```python
from build123d import *

# Parameters (mm, degrees)
F0_R     = 1
F0_R_2   = 0.5
F1_DEPTH = 4.2
F3_DEPTH = 3.2
F4_R     = 1.85
F4_R_2   = 1
F5_DEPTH = 2.2


with BuildPart() as f1:
    # F0 (on Top) → F1 (new body)
    with BuildSketch(Plane.XY):
        with BuildLine():
            Line((-1.99505, 12.940625), (-2.892823, 0.203906))
            ThreePointArc((-2.892823, 0.203906), (0, -2.9), (2.892823, 0.203906))
            Line((2.892823, 0.203906), (1.99505, 12.940625))
            ThreePointArc((1.99505, 12.940625), (0, 14.8), (-1.99505, 12.940625))
        make_face()
        Circle(F0_R, mode=Mode.SUBTRACT)
        with Locations((0, 4.8)):
            Circle(F0_R_2, mode=Mode.SUBTRACT)
        with Locations((0, 6.8)):
            Circle(F0_R_2, mode=Mode.SUBTRACT)
        with Locations((0, 8.8)):
            Circle(F0_R_2, mode=Mode.SUBTRACT)
        with Locations((0, 10.8)):
            Circle(F0_R_2, mode=Mode.SUBTRACT)
        with Locations((0, 12.8)):
            Circle(F0_R_2, mode=Mode.SUBTRACT)
    extrude(amount=F1_DEPTH)

    # F2 (on face) → F3 (cut)
    with BuildSketch(Plane(origin=(0, 0, 0), x_dir=(1, 0, 0), z_dir=(0, 0, -1))):
        with BuildLine():
            ThreePointArc((2.892823, -0.203906), (0, -2.9), (-2.892823, -0.203906))
            Line((-2.892823, -0.203906), (-1.99505, -12.940625))
            ThreePointArc((-1.99505, -12.940625), (0, -14.8), (1.99505, -12.940625))
            Line((1.99505, -12.940625), (2.892823, -0.203906))
        make_face()
    extrude(amount=-F3_DEPTH, mode=Mode.SUBTRACT)

    # F4 (on face) → F5 (cut)
    with BuildSketch(Plane(origin=(0, 0, 0), x_dir=(1, 0, 0), z_dir=(0, 0, -1))):
        Circle(F4_R)
        Circle(F4_R_2, mode=Mode.SUBTRACT)
    extrude(amount=-F5_DEPTH, mode=Mode.SUBTRACT)


solid = f1.part
```
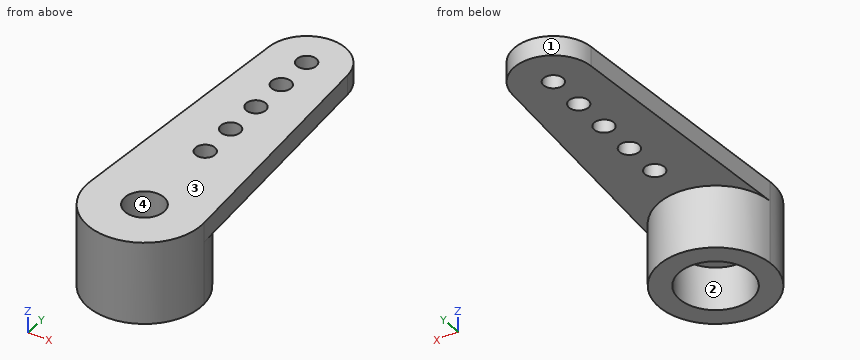
Work out the finished part from the listing and answer in its coordinate system (mm). Face numbers are marked on the shaded views. Round coordinates to 2 decimals unless told otherwise and drop trailing zeros. Loops run counter-clockwise (first coordinate to the right, second up) from the corner with the lowest first, then second, coordinate; pieces in that order, holes last. Notation, with made-up numbers: M 72,-26.75 L 123,-26.75 A30 ccw 123,-1.75 Z; hole C 82,-30 d2. An arc over 180 degrees is marked long. Use CSV: the item, a comma, the result in double quotes.
Q1. Section B-B, the plane x = 0.15 is taken. State how many separate pieces and enclosed holes the cut face has, then the cut area to 3 significant figures.
Determined:
separate pieces,"7"
enclosed holes,"0"
area,"19.4 mm2"
Q2. Section A-A, the plane y = 0 is taken. Determine the outline of the cut face in (x, z), then the cut area to 3 significant figures.
Determined:
outline,"M -2.9,0 L -1.85,0 L -1.85,2.2 L -1,2.2 L -1,4.2 L -2.9,4.2 Z; M 1,2.2 L 1.85,2.2 L 1.85,0 L 2.9,0 L 2.9,4.2 L 1,4.2 Z"
area,"12.2 mm2"
Q3. Section D-D, the plane y = 8.8 is taken. Determine the outline of the cut face in (x, z).
Determined:
outline,"M -2.29,3.2 L -0.5,3.2 L -0.5,4.2 L -2.29,4.2 Z; M 0.5,3.2 L 2.29,3.2 L 2.29,4.2 L 0.5,4.2 Z"
Q4. Each of these flat-tipped pins is pushed along its axis until it touches: pin 1 (2 mm diameter, centred on x = 2, y = 10, fed in from -Z); pin 2 (1 mm diameter, centred on y = 10, z = 3.5, fed in from +X). Where does it stop, or does it pass through?
Determined:
pin 1,"z = 3.2"
pin 2,"x = 2.24"
Q5. Section C-C, the plane z = 1.2 is taken. Determine the outline of the cut face in (x, y), then the cut area to 3 significant figures.
Determined:
outline,"C 0,0 d5.8; hole C 0,0 d3.7"
area,"15.7 mm2"
Q6. Consider L1, parallel to Z at x = -1.7, y = 8.25; L2, parallel to X at y = -1.25, z = 0.55; L3, parallel to X at y = 4.8, z = 3.55. Determine where each line is inside the solid, lowest interval first.
Determined:
L1,"3.2 to 4.2"
L2,"-2.62 to -1.36, 1.36 to 2.62"
L3,"-2.57 to -0.5, 0.5 to 2.57"
Q7. The mould has two halves that part along Y. Classify the marked faces 1, 2, 3 and 4: pulls with the +Y half, pulls with the -Y half, needs draft (parallel to the pull), parting line crosses it, or undercut.
Determined:
face 1,"pulls with the +Y half"
face 2,"undercut"
face 3,"needs draft"
face 4,"undercut"
